Work out the finished part from the listing and answer in its coordinate system (mm). Face numbers are marked on the shaded views. A direction names the side the tool comes from. Coordinates: 2 decimals unless noted, no trailing zeros. Order: outer loops, then holes, each group sorted by start corner. A loop starts at its lowest first (then second) coordinate and runs counter-clockwise, first axis right, second up.
1. The part is cut by section B-B, the plane y = 33. Give the vertices of the cut face in (x, z).
2. The part is cut by section D-D, the plane x = 475.5. Give the vertices of the cut face in (y, z).
3. Flat-ended cylindrical pins translate along their axes: pin 1 Ø8 at (x, y) = (401, 41) entering from +Z; pin 2 Ø12 at (y, z) = (34.5, 10.5) entering from -X; pin 3 Ø6 at (x, y) = (388.5, 42) entering from -Z; pin 4 Ø12 at (x, z) = (426.5, 15) entering from +Y. Find the tip coordinate at first contact, or state that the pin passes through.
4. The part is cut by section C-C, the plane z = 7.25. Give the vertices of the cut face in (x, y).
5. Find the intervals of material crossed by probe 1 along Y at (x, z) = (485.5, 4.75); probe 2 along X at (y, z) = (44, 1.5), in increasing order.
6. A tool of negligible diameter and unlimited length cuts with its end or side. For the marked faces 1 and 2, from which of +Z, -Z, +X, -X, +Y, -Y can it reach the whole face along a straight path? Write none if from no direction.
7. The part is cut by section A-A, the plane x = 409. Give the vertices of the cut face in (y, z).
Autodesk Inventor part; units mm, degrees
ref_plane "YZ Plane" through (0, 0, 0) normal (1, 0, 0) x (0, 1, 0)
ref_plane "XZ Plane" through (0, 0, 0) normal (0, 1, 0) x (-1, 0, 0)
ref_plane "XY Plane" through (0, 0, 0) normal (0, 0, 1) x (1, 0, 0)
sketch "Sketch1" plane through (0, 0, 0) normal (0, 0, 1) x (1, 0, 0)
  line L0 (-490, 54) -> (490, 54)
  line L1 (490, 54) -> (490, 0)
  line L2 (490, 0) -> (-490, 0)
  line L3 (-490, 0) -> (-490, 54)
  point P0 (0, 0)
  point P1 (0, 0)
  dimension "d0" = 980
  dimension "d1" = 54
extrude "Plate1" add sketch "Sketch1" along normal blind 2
sketch "Sketch2" plane through (490, 2, 0) normal (0, -1, 0) x (1, 0, 0)
  line L0 (-980, 0) -> (0, 0)
  line L1 (0, 0) -> (0, 20)
  line L2 (0, 20) -> (-980, 20)
  line L3 (-980, 20) -> (-980, 0)
edge flange "Flange1" height 20 angle 90 thickness 2 bend radius 2.75 thickness toward (0, -1, 0) relief round relief width 2 relief depth 1 edges at (0, 0, 2) wall of the first edge with corners at (-490, 2, 0) (490, 2, 0) (490, 2, 20) (-490, 2, 20)
bend "Bend1"
corner "Corner1"
sketch "Sketch5" plane through (0, 0, 0) normal (0, 0, -1) x (-1, 0, 0)
  line L0 (490, 54) -> (-490, 54)
  line L1 (490, 0) -> (-490, 0)
  circle A0 centre (0, 54) radius 35
  line L2 (243.95, 54) -> (246.05, 54)
  line L3 (246.05, 54) -> (246.05, 29)
  line L4 (246.05, 29) -> (243.95, 29)
  line L5 (243.95, 29) -> (243.95, 54)
  line L6 (-243.95, 54) -> (-246.05, 54)
  line L7 (-246.05, 54) -> (-246.05, 29)
  line L8 (-246.05, 29) -> (-243.95, 29)
  line L9 (-243.95, 29) -> (-243.95, 54)
  line L10 (0, 54) -> (0, 0) construction
  circle A1 centre (-490, 54) radius 35
  point P0 (0, 0)
  point P1 (245, 29)
  point P2 (-245, 29)
  point P3 (246.05, 54)
  point P4 (-35, 54)
  point P5 (35, 54)
  point P6 (-246.05, 54)
  dimension "d45" = 70
  dimension "d48" = 2.1
  dimension "d49" = 490
  dimension "d51" = 29
  dimension "d52" = 25
extrude "Extrusion1" cut sketch "Sketch5" against normal through all contours L3 L4 L5 L0 | L9 L8 L7 L0 | A0 L0 | A1 picked at (-5.9248, 35.8306)
sketch "Sketch9" plane through (0, 0, 2) normal (0, 0, 1) x (1, 0, 0)
  line L0 (485.6141, 29.596) -> (485.6141, 17.596) construction
  line L1 (485.6141, 17.596) -> (285.6141, 17.596) construction
  line L2 (285.6141, 17.596) -> (285.6141, 29.596) construction
  line L3 (285.6141, 29.596) -> (485.6141, 29.596) construction
  line L4 (-490, 54) -> (490, 54)
  point P0 (0, 0)
  point P1 (1.05, 68)
  point P2 (490, 54)
  dimension "d40" = 200
  dimension "d41" = 12
mark "Mark2"
sketch "Sketch10" plane through (-490, 0, 20) normal (0, -1, 0) x (1, 0, 0)
  line L0 (0, -20) -> (0, -18)
  line L1 (0, 0) -> (980, 0)
  line L2 (0, -20) -> (884.4148, -20)
  line L3 (884.4148, -20) -> (884.4148, 0)
  line L4 (884.4148, 0) -> (0, 0)
  line L5 (0, 0) -> (0, -20)
  line L6 (884.4148, 0) -> (860.5797, -20)
  point P0 (490, -20)
  dimension "d53" = 50
  dimension "d54" = 884.4148
extrude "Extrusion4" cut sketch "Sketch10" against normal through all contours L0 L5 L1 L6 L2
equation "\"d2\" = Thickness"
equation "\"d3\" = BendReliefWidth"
equation "\"d4\" = BendReliefDepth"
equation "\"d5\" = MinimumRemnant"
equation "\"d6\" = TransitionRadius"
equation "\"d9\" = BendRadius"
equation "\"d10\" = CornerReliefSize"
equation "\"d11\" = GapSize"
equation "\"d12\" = JacobiRadiusSize"
equation "\"BendReliefWidth\" = Thickness"
equation "\"BendReliefDepth\" = 0.5 * Thickness"
equation "\"CornerReliefSize\" = 4 * Thickness"
equation "\"MinimumRemnant\" = 2 * Thickness"
equation "\"TransitionRadius\" = BendRadius"
equation "\"JacobiRadiusSize\" = BendRadius"
equation "\"GapSize\" = Thickness"
properties part number "MSC 327 STRINGER BOARD  ###" material "Stainless Steel"
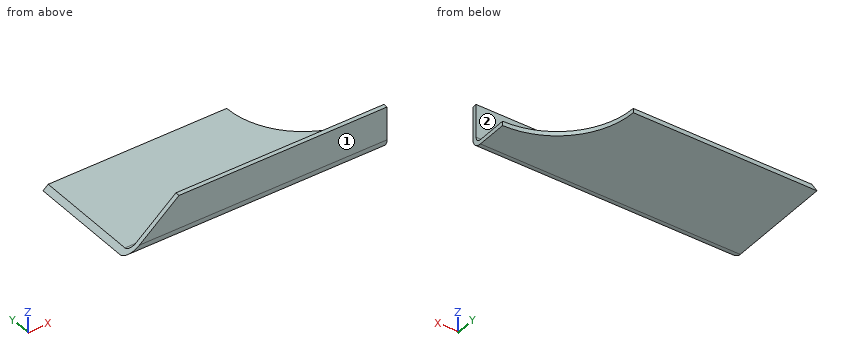
Geometry says:
1. outline: (370.58, 0) - (462, 0) - (462, 2) - (372.96, 2) - close
2. outline: (0, 4.75) arc R4.75 ccw to (4.75, 0) - (22.14, 0) - (22.14, 2) - (4.75, 2) arc R2.75 cw to (2, 4.75) - (2, 20) - (0, 20) - close
3. pin 1: stops at z = 2
3. pin 2: passes through
3. pin 3: stops at z = 0
3. pin 4: stops at y = 2
4. outline: (379.22, 0) - (490, 0) - (490, 2) - (379.22, 2) - close
5. probe 1: y = 0 to 2
5. probe 2: x = 372.37 to 456.46
6. face 1: +Z, -Z, +X, -X, -Y
6. face 2: +Z, +X, -X, +Y
7. outline: (0, 4.75) arc R4.75 ccw to (4.75, 0) - (54, 0) - (54, 2) - (4.75, 2) arc R2.75 cw to (2, 4.75) - (2, 20) - (0, 20) - close
